Geometry check sheet. Reference: the model listing, model coordinates, mm. A direction names the side the tool comes from. Coordinates: 2 decimals unless noted, no trailing zeros. Order: outer loops, then holes, each group sorted by start corner. A loop starts at its lowest first (then second) coordinate and runs counter-clockwise, first axis right, second up.
Autodesk Inventor part; units mm, degrees
ref_plane "Work Plane1" through (0, 0, 29) normal (0, 0, -1) x (-1, 0, 0)
ref_plane "YZ Plane" through (0, 0, 0) normal (1, 0, 0) x (0, 1, 0)
ref_plane "XZ Plane" through (0, 0, 0) normal (0, 1, 0) x (-1, 0, 0)
sketch "Sketch1" plane through (0, 0, 0) normal (0, 0, 1) x (1, 0, 0)
  circle A0 centre (0, 0) radius 11
  dimension "d0" = 22
extrude "Extrusion1" add sketch "Sketch1" along normal blind 60
sketch "Sketch2" plane through (0, 0, 60) normal (0, 0, 1) x (1, 0, 0)
  circle A0 centre (0, 0) radius 2
  dimension "d3" = 4
extrude "Extrusion2" add sketch "Sketch2" along normal blind 15
ref_plane "Work Plane1" through (0, 0, 29) normal (0, 0, -1) x (-1, 0, 0)
sketch "Sketch3" plane through (0, 0, 29) normal (0, 0, -1) x (-1, 0, 0)
  line L0 (16.5, -18) -> (-16.5, -18) construction
  line L1 (-16.5, -18) -> (-16.5, 18) construction
  line L2 (-16.5, 18) -> (16.5, 18) construction
  line L3 (16.5, 18) -> (16.5, -18) construction
  line L4 (16.5, -18) -> (-16.5, 18) construction
  line L5 (-16.5, -18) -> (16.5, 18) construction
  arc A0 (-13.4629, -1) -> (13.4629, -1) centre (0, 0) ccw construction
  circle A1 centre (0, 0) radius 13.5
  line L6 (16.5, 18) -> (-16.5, 18)
  line L7 (-16.5, 18) -> (-16.5, -1)
  line L8 (-16.5, -1) -> (16.5, -1)
  line L9 (16.5, -1) -> (16.5, 18)
  dimension "d7" = 33
  dimension "d8" = 36
  dimension "d9" = 27
  dimension "d10" = 27
  dimension "d11" = 19
extrude "Extrusion3" add sketch "Sketch3" against normal blind 6.5
sketch "Sketch4" plane through (-16.5, 18, 29) normal (0, 1, 0) x (1, 0, 0)
  line L0 (3.0371, 0) -> (0, 0) construction
  line L1 (0, 0) -> (33, 0) construction
  line L2 (33, 0) -> (33, -3.25) construction
  line L3 (33, -3.25) -> (0, -3.25) construction
  line L4 (0, -3.25) -> (0, 0) construction
  line L5 (0, -3.25) -> (3, -3.25) construction
  line L6 (33, -3.25) -> (30, -3.25) construction
  circle A0 centre (3, -3.25) radius 1.75
  circle A1 centre (30, -3.25) radius 1.75
  point P0 (16.5, 29)
  dimension "d14" = 33
  dimension "d15" = 3.25
  dimension "d16" = 3
  dimension "d17" = 3
  dimension "d18" = 3.5
  dimension "d19" = 3.5
extrude "Extrusion4" cut sketch "Sketch4" against normal blind 5
properties part number "Small Motor"
Item 1: Release check for a two-part mould opening along Z. For faces 6 (the face through (0.283, -13.497, 32.205)), 7 (the face through (0, 13, 29)), 8 (the face through (-14, 13, 32)) record: pulls with the +Z half, pulls with the -Z half, needs draft (parallel to the pull), parting line crosses it, or undercut.
Item 2: Thickness scan on line 1 along X through (y, z) = (16, 32); line 2 along Z through (x, y) = (13.5, 17); line 3 along Z through (x, y) = (0, -8.5). Record the ranges inside material, lowest first.
Item 3: Sectioned sample at C-C (y = 0). Record the cut outline in (x, z), and give its area (3 significant figures).
Item 4: Sectioned sample at B-B (x = 0). Record the cut outline in (y, z).
Item 5: Depth check by flat-ended pin: P1, Ø3.5, axis at x = 14, z = 31.5, coming from the -Y side; P2, Ø1, axis at x = -6, y = 14.5, coming from the -Z side; P3, Ø2, axis at x = -10, y = 14, coming from the +Z side. Enter the tip coordinate at first touch or a pass-through.
Item 6: Sectioned sample at D-D (x = -5). Record the cut outline in (y, z), and give its area (3 significant figures).
Item 7: Sectioned sample at A-A (z = 32.25). Record the cut outline in (x, y).
Item 8: Tool access check on faces 1 (the face through (-15, -1, 32)), 2 (the face through (15.169, 15.535, 31.724)), 3 (the face through (15, -1, 32)), 4 (the face through (0, 13, 35.5)), 5 (the face through (-2.38, 10.74, 14.3)). Record the directions out of +Z, -Z, +X, -X, +Y, -Y that give a thin tool (end or side, any length) a straight path to the whole face; none if there is none.
Geometry check:
1. face 6: needs draft
1. face 7: pulls with the -Z half
1. face 8: undercut
2. line 1: x = -16.5 to -15.23, -11.77 to 11.77, 15.23 to 16.5
2. line 2: z = 29 to 30.5, 34 to 35.5
2. line 3: z = 0 to 60
3. outline: (-16.5, 29) - (-11, 29) - (-11, 0) - (11, 0) - (11, 29) - (16.5, 29) - (16.5, 35.5) - (11, 35.5) - (11, 60) - (2, 60) - (2, 75) - (-2, 75) - (-2, 60) - (-11, 60) - (-11, 35.5) - (-16.5, 35.5) - close
3. area: 1,450 mm2
4. outline: (-13.5, 29) - (-11, 29) - (-11, 0) - (11, 0) - (11, 29) - (18, 29) - (18, 35.5) - (11, 35.5) - (11, 60) - (2, 60) - (2, 75) - (-2, 75) - (-2, 60) - (-11, 60) - (-11, 35.5) - (-13.5, 35.5) - close
5. P1: stops at y = -5.67
5. P2: stops at z = 29
5. P3: stops at z = 35.5
6. outline: (-12.54, 29) - (-9.8, 29) - (-9.8, 0) - (9.8, 0) - (9.8, 29) - (18, 29) - (18, 35.5) - (9.8, 35.5) - (9.8, 60) - (-9.8, 60) - (-9.8, 35.5) - (-12.54, 35.5) - close
6. area: 1,250 mm2
7. outline: (-16.5, -1) - (-13.46, -1) arc R13.5 ccw to (13.46, -1) - (16.5, -1) - (16.5, 18) - (15.25, 18) - (15.25, 13) - (11.75, 13) - (11.75, 18) - (-11.75, 18) - (-11.75, 13) - (-15.25, 13) - (-15.25, 18) - (-16.5, 18) - close
8. face 1: +Z, -Z, -X, -Y
8. face 2: +Y
8. face 3: +Z, -Z, +X, -Y
8. face 4: +Z
8. face 5: -Z
